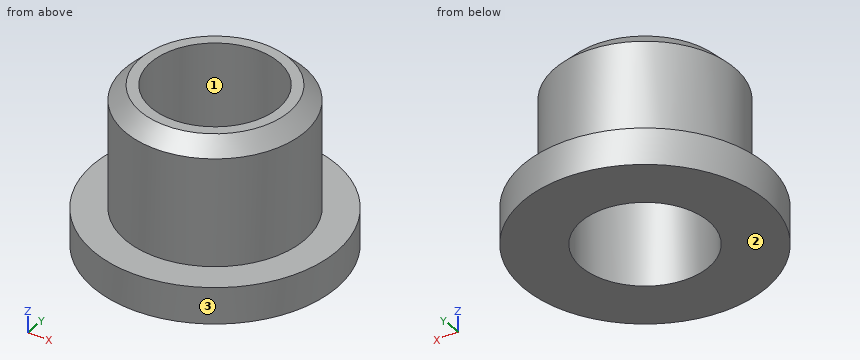
Autodesk Inventor part; units mm, degrees
ref_plane "YZ Plane" through (0, 0, 0) normal (1, 0, 0) x (0, 1, 0)
ref_plane "XZ Plane" through (0, 0, 0) normal (0, 1, 0) x (-1, 0, 0)
ref_plane "XY Plane" through (0, 0, 0) normal (0, 0, 1) x (1, 0, 0)
sketch "Эскиз1" plane through (0, 0, 0) normal (0, 0, 1) x (1, 0, 0)
  circle A0 centre (0, 0) radius 2.95
  circle A1 centre (0, 0) radius 2.1
  circle A2 centre (0, 0) radius 4
  dimension "d0" = 5.9
  dimension "d1" = 4.2
  dimension "d2" = 8
sketch "Эскиз2" plane through (0, 0, 0) normal (0, 0, 1) x (1, 0, 0)
  circle A0 centre (0, 0) radius 2.95
  circle A1 centre (0, 0) radius 2.1
  circle A2 centre (0, 0) radius 4
extrude "Выдавливание1" add sketch "Эскиз2" along normal blind 1.2 contours A0 | A2
sketch "Эскиз4" plane through (0, 0, 1.2) normal (0, 0, 1) x (1, 0, 0)
  circle A0 centre (0, 0) radius 2.95
  circle A1 centre (0, 0) radius 2.1
  dimension "d7" = 5.9
extrude "Выдавливание3" add sketch "Эскиз4" along normal blind 4.05
chamfer "Фаска1" distance 0.5 angle 45 1 edges at (-2.95, 0, 5.25)
properties part number "middle_gear_fixator"
Geometry check sheet. Reference: the model listing, model coordinates, mm. Face numbers are marked on the shaded views. Round coordinates to 2 decimals unless told otherwise and drop trailing zeros. Loops run counter-clockwise (first coordinate to the right, second up) from the corner with the lowest first, then second, coordinate; pieces in that order, holes last. Notation, with made-up numbers: M -6.5,-2 L 10.5,-2 A13 ccw 10.5,14 Z; hole C 82.5,51 d8. An arc over 180 degrees is marked long. Return JSON: item names as keys, results as strings. Group by question number.
(1) Section check A-A, the plane y = 0. Enter the section's corners in (x, z).
(2) Scan lines: line 1 along Y through (x, z) = (0, 3.6); line 2 along Z through (x, y) = (-3.25, -0.5); line 3 along X through (y, z) = (0.25, 2.9). Record each from-to range of solid material in increasing order. Write a range as [from, to].
(3) Mould release check, pull along Y, two halves, no side actions. Record for the marked faces 1, 2 and 3: pulls with the +Y half, pulls with the -Y half, needs draft (parallel to the pull), parting line crosses it, or undercut.
(4) Section check C-C, the plane z = 4.65. Enter the section's corners in (x, y), and give its area (3 significant figures).
(5) Go/stop test with flat-tipped pins: pin 1 (3 mm diameter, centred on y = 0, z = 4, fed in from -X); pin 2 (2 mm diameter, centred on y = -1, z = 4.5, fed in from -X); pin 3 (2 mm diameter, centred on x = 2.5, z = 4.5, fed in from -Y). Record where each tip stops, or that it passes through.
(6) Section check D-D, the plane y = 3.75. Enter the section's corners in (x, z).
Data:
{
 "1": {"outline": "M -4,0 L -2.1,0 L -2.1,5.25 L -2.45,5.25 L -2.95,4.75 L -2.95,1.2 L -4,1.2 Z; M 2.1,0 L 4,0 L 4,1.2 L 2.95,1.2 L 2.95,4.75 L 2.45,5.25 L 2.1,5.25 Z"},
 "2": {"line 1": "[-2.95, -2.1], [2.1, 2.95]", "line 2": "[0, 1.2]", "line 3": "[-2.94, -2.09], [2.09, 2.94]"},
 "3": {"face 1": "undercut", "face 2": "needs draft", "face 3": "parting line crosses it"},
 "4": {"outline": "C 0,0 d5.9; hole C 0,0 d4.2", "area": "13.5 mm²"},
 "5": {"pin 1": "x = -2.95", "pin 2": "x = -2.95", "pin 3": "y = -2.54"},
 "6": {"outline": "M -1.39,0 L 1.39,0 L 1.39,1.2 L -1.39,1.2 Z"}
}
